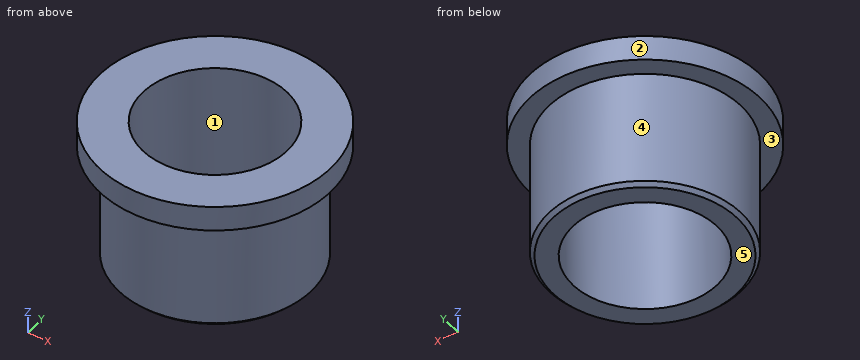
```python
from build123d import *

# Parameters (mm, degrees)
F_1_4_0_75_DIAMETER_HOLE1_D = 19.05
CHAMFER2_SIZE               = 0.508


with BuildPart() as part:
    # Sketch2 → Revolve2 (revolve)
    with BuildSketch(Plane(origin=(0, 0, 0), x_dir=(0, 0, -1), z_dir=(1, 0, 0))):
        Polygon((0, 0), (-18.8214, 0), (-18.8214, 15.244233333), (-15.5194, 15.244233333), (-15.5194, 12.7), (0, 12.7), align=None)
    revolve(axis=Axis((0, 0, 0), (0, 0, -1)))

    # 1/4 (0.75) Diameter Hole1 (through all)
    with Locations(Plane.XY.offset(18.8214)):
        with Locations((0, 0)):
            Hole(F_1_4_0_75_DIAMETER_HOLE1_D / 2)

    # Chamfer2
    chamfer2_edges = [part.edges().sort_by_distance(p)[0] for p in [
        (0, -12.7, 0),
    ]]
    chamfer(chamfer2_edges, length=CHAMFER2_SIZE)


solid = part.part
```
Verification items for the finished model (mm, model axes). Face numbers are marked on the shaded views. A direction names the side the tool comes from. Round coordinates to 2 decimals unless told otherwise and drop trailing zeros. Order: outer loops, then holes, each group sorted by start corner. A loop starts at its lowest first (then second) coordinate and runs counter-clockwise, first axis right, second up. Notation, with made-up numbers: (6, 59.5) -> (64, 59.5) arc R13 cw to (64, 84.5) -> close; hole circle Ø3 at (22, 70). An arc over 180 degrees is marked (long way). Put each result on its own line as item: value. Start each with the question number.
(1) Tool access check on the marked faces 4 and 5. Record the directions out of +Z, -Z, +X, -X, +Y, -Y that give a thin tool (end or side, any length) a straight path to the whole face; none if there is none.
(2) Depth check by flat-ended pin: pin 1 Ø2 at (y, z) = (-6.5, 4) entering from -X; pin 2 Ø3 at (y, z) = (-3.5, 9) entering from +X; pin 3 Ø8 at (x, z) = (9.5, 4.5) entering from -Y. Enter the tip coordinate at first touch or a pass-through.
(3) Section check C-C (z = 16.75). Enter the section's corners in (x, y) (3 decimals), then the cut area to 3 significant figures.
(4) Section check D-D (z = 10.5). Enter the section's corners in (x, y) (3 decimals), then the cut area to 3 significant figures.
(5) Material ranges on line 1 along X through (y, z) = (-8, 8.75); line 2 along Y through (x, z) = (7, 5); line 3 along Y through (x, z) = (-1, 17.25), recorded low to high.
(6) Section check A-A (y = 0). Enter the section's corners in (x, z) (3 decimals).
(7) Draft check along X on the marked faces 1, 2 and 3. Enter one of: +X half, -X half, draft (parallel to the pull), parting line (faces both ways), or undercut.
Completed:
1. face 4: -Z
1. face 5: -Z, +X, -X, +Y, -Y
2. pin 1: stops at x = -11.45
2. pin 2: stops at x = 12.54
2. pin 3: stops at y = -11.45
3. outline: circle Ø30.488 at (0, 0); hole circle Ø19.05 at (0, 0)
3. area: 445 mm2
4. outline: circle Ø25.4 at (0, 0); hole circle Ø19.05 at (0, 0)
4. area: 222 mm2
5. line 1: x = -9.86 to -5.17, 5.17 to 9.86
5. line 2: y = -10.6 to -6.46, 6.46 to 10.6
5. line 3: y = -15.21 to -9.47, 9.47 to 15.21
6. outline: (-15.244, 15.519) -> (-12.7, 15.519) -> (-12.7, 0.508) -> (-12.192, 0) -> (-9.525, 0) -> (-9.525, 18.821) -> (-15.244, 18.821) -> close; (9.525, 0) -> (12.192, 0) -> (12.7, 0.508) -> (12.7, 15.519) -> (15.244, 15.519) -> (15.244, 18.821) -> (9.525, 18.821) -> close
7. face 1: undercut
7. face 2: parting line
7. face 3: draft
